from build123d import *

# Parameters (mm, degrees)
F1_DEPTH = 7.5
F2_DEPTH = 4.7
F3_R     = 5
F4_R     = 3
F5_DEPTH = 25


with BuildPart() as f1:
    # F0 (on Front) → F1 (new body)
    with BuildSketch(Plane.XZ):
        with BuildLine():
            Line((-40.22098, 7.35), (0, 7.35))
            Line((0, 7.35), (0, 15))
            Line((0, 15), (-40, 15))
            ThreePointArc((-40, 15), (-55, 0), (-40, -15))
            Line((-40, -15), (0, -15))
            Line((0, -15), (0, -7.35))
            Line((0, -7.35), (-40.22098, -7.35))
            ThreePointArc((-40.22098, -7.35), (-47.57098, 0), (-40.22098, 7.35))
        make_face()
    extrude(amount=F1_DEPTH)

    # F0 (on Front) → F2 (join)
    with BuildSketch(Plane.XZ):
        with BuildLine():
            ThreePointArc((0, -7.35), (-7.35, 0), (0, 7.35))
            Line((0, 7.35), (-40.22098, 7.35))
            ThreePointArc((-40.22098, 7.35), (-35.023746, 5.197235), (-32.87098, 0))
            ThreePointArc((-32.87098, 0), (-35.023746, -5.197235), (-40.22098, -7.35))
            Line((-40.22098, -7.35), (0, -7.35))
        make_face()
        with BuildLine():
            ThreePointArc((-32.87098, 0), (-35.023746, 5.197235), (-40.22098, 7.35))
            ThreePointArc((-40.22098, 7.35), (-47.57098, 0), (-40.22098, -7.35))
            ThreePointArc((-40.22098, -7.35), (-35.023746, -5.197235), (-32.87098, 0))
        make_face()
        with BuildLine():
            ThreePointArc((0, -7.35), (5.197235, -5.197235), (7.35, 0))
            ThreePointArc((7.35, 0), (5.197235, 5.197235), (0, 7.35))
            Line((0, 7.35), (0, 0))
            Line((0, 0), (0, -7.35))
        make_face()
        with BuildLine():
            Line((0, 0), (0, 7.35))
            ThreePointArc((0, 7.35), (-7.35, 0), (0, -7.35))
            Line((0, -7.35), (0, 0))
        make_face()
    extrude(amount=F2_DEPTH)

    # F3
    f3_edges = [f1.edges().sort_by_distance(p)[0] for p in [
        (-20, -7.5, 15),
    ]]
    fillet(f3_edges, radius=F3_R)

    # F4 (on face) → F5 (cut)
    with BuildSketch(Plane.XZ.offset(4.7)):
        with Locations((-40.22098, 0)):
            Circle(F4_R)
    extrude(amount=-F5_DEPTH, mode=Mode.SUBTRACT)


solid = f1.part
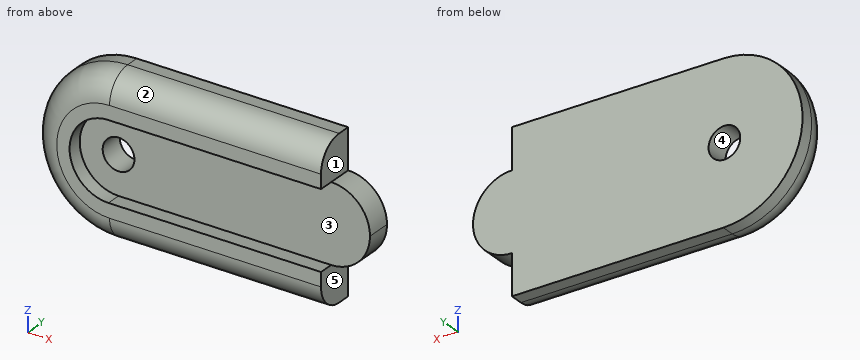
Input: part model. Units: mm. Frame: model coordinates. Face numbers are marked on the shaded views. A direction names the side the tool comes from. Coordinates: 2 decimals unless noted, no trailing zeros. Loops run counter-clockwise (first coordinate to the right, second up) from the corner with the lowest first, then second, coordinate; pieces in that order, holes last.
Q1. Set-up query: the marked faces 1 and 2. Return all of +Z, -Z, +X, -X, +Y, -Y with unobstructed straight access to the full face (end or side cutting, diameter ignored); none if empty.
Q2. Cut plane A-A (y = -1.75). Output: boundary loops of the cut face in (x, z), then the cut area to 3 significant figures.
Q3. Draft query along X for the marked faces 3, 4 and 5. Return one class per face: +X half, -X half, draft (parallel to the pull), parting line (faces both ways), or undercut.
Q4. Cut plane B-B (x = -31). Output: boundary loops of the cut face in (y, z).
Q5. Material intervals for line 1 (Y direction, x = -0.5, z = 2.5); line 2 (Z direction, x = -16, y = -6.75); line 3 (Z direction, x = -38.5, y = -3), sorted ascending.
Q6. Contact query for flat-ended pins moving along their axis: pin 1 (0.8 mm diameter, centred on x = -13, y = -6.5, fed in from -Z); pin 2 (2 mm diameter, centred on x = -20.5, y = -5.5, fed in from +Z); pin 3 (2 mm diameter, centred on y = -4, z = -11, fed in from +X). Output: stop coordinate, or through.
Working result:
1. face 1: +Z, +X, +Y, -Y
1. face 2: +Z, +X, -X, -Y
2. outline: (-40, -15) - (0, -15) - (0, -7.35) arc R7.35 ccw to (7.35, 0) arc R7.35 ccw to (0, 7.35) - (0, 15) - (-40, 15) arc R15 ccw to start; hole circle Ø6 at (-40.22, 0)
2. area: 1,610 mm2
3. face 3: draft
3. face 4: undercut
3. face 5: +X half
4. outline: (-7.5, -10) arc R5 ccw to (-2.5, -15) - (0, -15) - (0, 15) - (-2.5, 15) arc R5 ccw to (-7.5, 10) - (-7.5, 7.35) - (-4.7, 7.35) - (-4.7, -7.35) - (-7.5, -7.35) - close
5. line 1: y = -4.7 to 0
5. line 2: z = -12.63 to -7.35, 7.35 to 12.63
5. line 3: z = -14.97 to -2.46, 2.46 to 14.97
6. pin 1: stops at z = -13.47
6. pin 2: stops at z = 14.58
6. pin 3: stops at x = 0
